For this review, take the finished solid that the model builds, in its own axes (mm). Coordinates: 2 decimals unless noted, no trailing zeros. Loops run counter-clockwise (first coordinate to the right, second up) from the corner with the lowest first, then second, coordinate; pieces in that order, holes last. Notation, with made-up numbers: (-35.5, 16.25) -> (9.5, 16.25) arc R23 cw to (9.5, 31.25) -> close; hole circle Ø10 at (56.5, 28). An arc over 180 degrees is marked (long way). Answer in a Markdown table with one row per item.
from build123d import *

# Parameters (mm, degrees)
SKETCH1_R               = 49.53
SKETCH1_R_2             = 47.9425
BOSS_EXTRUDE1_DEPTH     = 152.4
CUT_EXTRUDE1_DEPTH      = 642.495475246
CUT_EXTRUDE1_DEPTH_BACK = 642.495475246
SKETCH2_R               = 1.905


with BuildPart() as part:
    # Sketch1 → Boss-Extrude1 (new body)
    with BuildSketch(Plane(origin=(0, 0, 0), x_dir=(0, 0, -1), z_dir=(1, 0, 0))):
        with Locations(Location((0, 0, 0), (0, 0, 180))):
            Circle(SKETCH1_R)
        with Locations(Location((0, 0, 0), (0, 0, 180))):
            Circle(SKETCH1_R_2, mode=Mode.SUBTRACT)
    extrude(amount=BOSS_EXTRUDE1_DEPTH)

    # Sketch2 → Cut-Extrude1 (cut, two sides: drawn at the far end of the back side and taken through both)
    with BuildSketch(Plane(origin=(-485.259786219, 0, 0), x_dir=(0, 0.12524438136346008, 0.9921259219156024), z_dir=(0, 0.9921259219156026, -0.12524438136346008)).offset(-CUT_EXTRUDE1_DEPTH_BACK)):
        with Locations((12.7, 501.801536219)):
            Circle(SKETCH2_R)
        with Locations((0, 501.801536219)):
            Circle(SKETCH2_R)
        with Locations((-12.7, 501.801536219)):
            Circle(SKETCH2_R)
    extrude(amount=CUT_EXTRUDE1_DEPTH + CUT_EXTRUDE1_DEPTH_BACK, mode=Mode.SUBTRACT)


solid = part.part
Item 1: Take a section at C-C, the plane x = 46. State the section outline as (y, z) points (1 decimal).
Worked answers:
| item | result |
|---|---|
| outline | circle Ø99.1 at (0, 0); hole circle Ø95.9 at (0, 0) |
Item 2: Take a section at A-A, the plane y = 0. State the section outline as (x, z) points.
Worked answers:
| item | result |
|---|---|
| outline | (0, -49.53) -> (152.4, -49.53) -> (152.4, -47.94) -> (0, -47.94) -> close; (0, 47.94) -> (152.4, 47.94) -> (152.4, 49.53) -> (0, 49.53) -> close |
Item 3: For L1, parallel to Y at x = 72, z = 0; L2, parallel to Y at x = 41, z = 21.5; L3, parallel to Z at x = 138, y = 33, list the stretches that pass through material, from the lowest coordinate up.
Worked answers:
| item | result |
|---|---|
| L1 | -49.53 to -47.94, 47.94 to 49.53 |
| L2 | -44.62 to -42.85, 42.85 to 44.62 |
| L3 | -36.94 to -34.78, 34.78 to 36.94 |
Item 4: The part is to be moulded in two halves that separate along X. For faces 1 (the flat face through (152.4, -41, -26)), 2 (the flat face through (0, -41, -26)), 3 (the cylindrical face through (15.81, 48.43, 8.46)), say which applies: +X half, -X half, draft (parallel to the pull), parting line (faces both ways), or undercut.
Worked answers:
| item | result |
|---|---|
| face 1 | +X half |
| face 2 | -X half |
| face 3 | undercut |
Item 5: Insertion check: pin 1 (12 mm diameter, centred on x = 115, z = -10, fed in from -Y); pin 2 (4 mm diameter, centred on x = 116.5, y = -3.5, fed in from -Z); pin 3 (6 mm diameter, centred on x = 76.5, z = -13, fed in from -Y). Each pin has a flat end and moves straight along its axis. Give the tip position at first contact, or say it passes through.
Worked answers:
| item | result |
|---|---|
| pin 1 | y = -49.37 |
| pin 2 | z = -49.51 |
| pin 3 | y = -48.51 |
